Source: three-view drawing plus pictorial views. Frame: mm from the lowest corner of the part. Give positions to 0.01 mm unless a question says otherwise; leave off trailing zeros. Write each loop counter-clockwise with the first axis right and the second up, starting at its lowest first coordinate (ties: lowest second). Pieces come first, ordered by that corner, then holes.
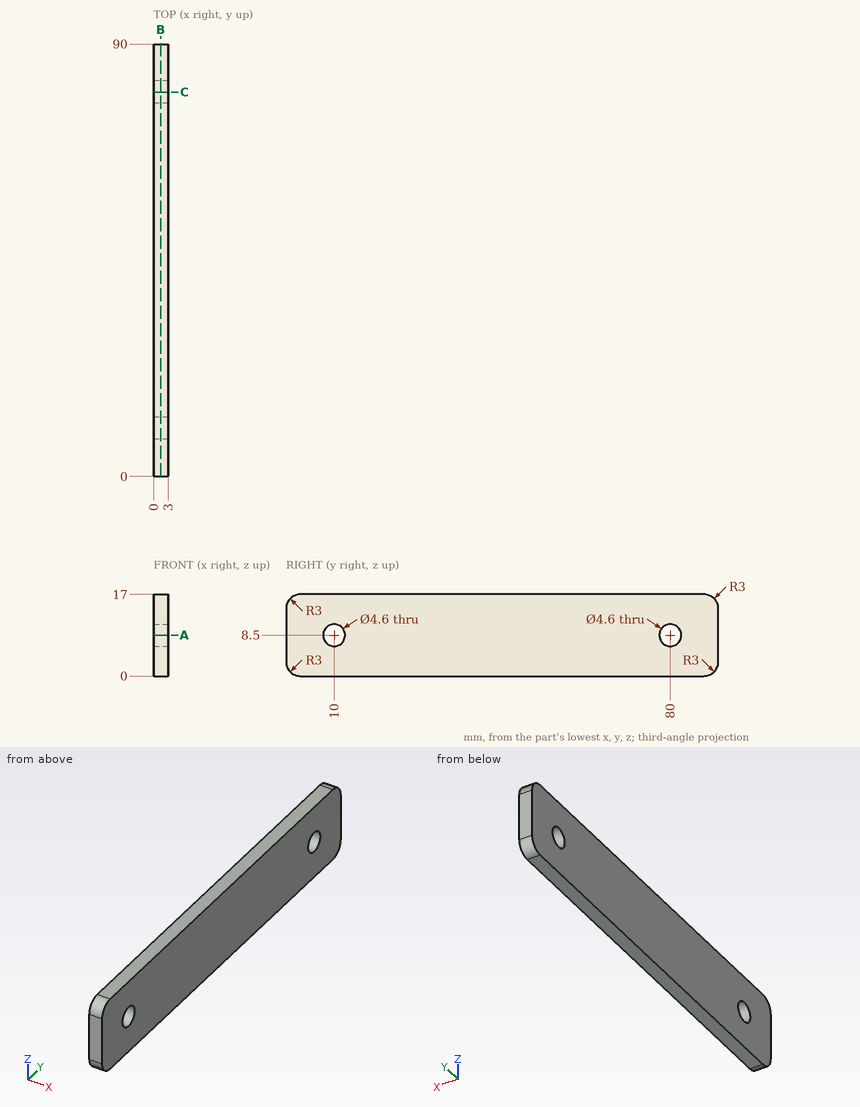
Q1. Section B-B on x = 1.45. Output: boundary loops of the cut face in (y, z), plus the area to 3 significant figures.
Filled sheet:
outline: (0, 3) arc R3 ccw to (3, 0) - (87, 0) arc R3 ccw to (90, 3) - (90, 14) arc R3 ccw to (87, 17) - (3, 17) arc R3 ccw to (0, 14) - close; hole circle Ø4.6 at (10, 8.5); hole circle Ø4.6 at (80, 8.5)
area: 1,490 mm2
Q2. Pin query (flat end, axial travel): P1, Ø1.5, axis at x = 2, z = 15, coming from the +Y side; P2, Ø4, axis at y = 80, z = 8.5, coming from the -X side. Return the tip coordinate at first contact, or that it passes through.
Filled sheet:
P1: stops at y = 89.99
P2: passes through
Q3. Ray query, line 1 along Y through (x, z) = (1.9, 8.5); line 2 along Z through (x, y) = (2.45, 80); line 3 along Y through (x, z) = (1.1, 7). Return the intervals inside material, ascending.
Filled sheet:
line 1: y = 0 to 7.7, 12.3 to 77.7, 82.3 to 90
line 2: z = 0 to 6.2, 10.8 to 17
line 3: y = 0 to 8.26, 11.74 to 78.26, 81.74 to 90
Q4. Section C-C on y = 80. Output: boundary loops of the cut face in (x, z).
Filled sheet:
outline: (0, 0) - (3, 0) - (3, 6.2) - (0, 6.2) - close; (0, 10.8) - (3, 10.8) - (3, 17) - (0, 17) - close
Q5. Section A-A on z = 8.5. Output: boundary loops of the cut face in (x, y), plus the area to 3 significant figures.
Filled sheet:
outline: (0, 0) - (3, 0) - (3, 7.7) - (0, 7.7) - close; (0, 12.3) - (3, 12.3) - (3, 77.7) - (0, 77.7) - close; (0, 82.3) - (3, 82.3) - (3, 90) - (0, 90) - close
area: 242 mm2
